Could you check a few things on this model? Use its own coordinates, in mm. A direction names the side the tool comes from. Round coordinates to 2 decimals unless told otherwise and drop trailing zeros. Loops run counter-clockwise (first coordinate to the right, second up) from the corner with the lowest first, then second, coordinate; pieces in that order, holes last. Notation, with made-up numbers: (-37, 49) -> (-30, 49) arc R12 ccw to (-30, 68) -> close; hole circle Ø6 at (-13, 11). An arc over 180 degrees is marked (long way). One line per item, written item: value.
from build123d import *

# Parameters (mm, degrees)
SKETCH1_R                  = 1.1
SKETCH1_W                  = 3
SKETCH1_H                  = 5
SKETCH1_W_2                = 6
SKETCH1_H_2                = 8
BOSS_EXTRUDE1_DEPTH        = 6
F_1_6_1_6_DIAMETER_HOLE3_D = 1.6
BOSS_EXTRUDE2_DEPTH        = 6
FILLET1_R                  = 2
F_2_2_2_2_DIAMETER_HOLE1_D = 2.2
F_4_0MM_DOWEL_HOLE1_D      = 4.5


with BuildPart() as part:
    # Sketch1 → Boss-Extrude1 (new body)
    with BuildSketch(Plane(origin=(0, 0, 0), x_dir=(1, 0, 0), z_dir=(0, 1, 0))):
        Polygon((14.366669751, 50.883801944), (36.883330249, 37.883801944), (36.883330249, -37.883801944), (14.366669751, -50.883801944), (5.706415713, -45.883801944), (5.706415713, -28), (-25.269237886, -28), (-51.25, -13), (-51.25, 13), (-25.269237886, 28), (5.706415713, 28), (5.706415713, 45.883801944), align=None)
        with Locations(Location((14.205771366, 42.605117767, 0), (0, 0, 270))):
            Circle(SKETCH1_R, mode=Mode.SUBTRACT)
        with Locations(Location((29.794228634, 33.605117767, 0), (0, 0, 270))):
            Circle(SKETCH1_R, mode=Mode.SUBTRACT)
        with Locations(Location((29.794228634, -33.605117767, 0), (0, 0, 270))):
            Circle(SKETCH1_R, mode=Mode.SUBTRACT)
        with Locations(Location((14.205771366, -42.605117767, 0), (0, 0, 270))):
            Circle(SKETCH1_R, mode=Mode.SUBTRACT)
        with Locations(Location((-44, 9, 0), (0, 0, 270))):
            Circle(SKETCH1_R, mode=Mode.SUBTRACT)
        with Locations(Location((-44, -9, 0), (0, 0, 270))):
            Circle(SKETCH1_R, mode=Mode.SUBTRACT)
        with BuildLine():
            Line((4.75, -20), (-15.25, -20))
            Line((-15.25, -20), (-15.25, -22))
            Line((-15.25, -22), (-27.25, -22))
            ThreePointArc((-27.25, -22), (-29.75, -19.5), (-27.25, -17))
            Line((-27.25, -17), (-17.25, -17))
            Line((-17.25, -17), (-17.25, 20))
            Line((-17.25, 20), (4.75, 20))
            Line((4.75, 20), (4.75, -20))
        make_face(mode=Mode.SUBTRACT)
        Polygon((30.071152423, 40.084763838), (34.401279442, 37.584763838), (32.901279442, 34.986687627), (28.571152423, 37.486687627), align=None, mode=Mode.SUBTRACT)
        Polygon((15.348720558, 48.584763838), (13.848720558, 45.986687627), (18.178847577, 43.486687627), (19.678847577, 46.084763838), align=None, mode=Mode.SUBTRACT)
        Polygon((34.401279442, -37.584763838), (32.901279442, -34.986687627), (28.571152423, -37.486687627), (30.071152423, -40.084763838), align=None, mode=Mode.SUBTRACT)
        Polygon((18.178847577, -43.486687627), (19.678847577, -46.084763838), (15.348720558, -48.584763838), (13.848720558, -45.986687627), align=None, mode=Mode.SUBTRACT)
        with Locations((-48.25, -8.5)):
            Rectangle(SKETCH1_W, SKETCH1_H, mode=Mode.SUBTRACT)
        with Locations((-48.25, 8.5)):
            Rectangle(SKETCH1_W, SKETCH1_H, mode=Mode.SUBTRACT)
        with BuildLine():
            Line((-30.75, 14.5), (-30.75, 17.5))
            ThreePointArc((-30.75, 17.5), (-29.25, 19), (-27.75, 17.5))
            Line((-27.75, 17.5), (-27.75, 14.5))
            ThreePointArc((-27.75, 14.5), (-29.25, 13), (-30.75, 14.5))
        make_face(mode=Mode.SUBTRACT)
        with BuildLine():
            Line((24.206415713, -25), (24.206415713, -22))
            ThreePointArc((24.206415713, -22), (25.706415713, -20.5), (27.206415713, -22))
            Line((27.206415713, -22), (27.206415713, -25))
            ThreePointArc((27.206415713, -25), (25.706415713, -26.5), (24.206415713, -25))
        make_face(mode=Mode.SUBTRACT)
        with BuildLine():
            Line((24.206415713, 22), (24.206415713, 25))
            ThreePointArc((24.206415713, 25), (25.706415713, 26.5), (27.206415713, 25))
            Line((27.206415713, 25), (27.206415713, 22))
            ThreePointArc((27.206415713, 22), (25.706415713, 20.5), (24.206415713, 22))
        make_face(mode=Mode.SUBTRACT)
        with Locations((29.633330249, 0)):
            Rectangle(SKETCH1_W_2, SKETCH1_H_2, mode=Mode.SUBTRACT)
    extrude(amount=BOSS_EXTRUDE1_DEPTH)

    # Ø1.6 (1.6) Diameter Hole3 (through all)
    with Locations(Plane(origin=(-6.25, 0, 22.5), x_dir=(0, 0, -1), z_dir=(0, -1, 0))):
        with Locations((0, 0), (45, 0)):
            Hole(F_1_6_1_6_DIAMETER_HOLE3_D / 2)

    # Sketch9 → Boss-Extrude2 (add)
    with BuildSketch(Plane.XZ):
        with BuildLine():
            Line((36.883330249, -9), (36.883330249, -15))
            ThreePointArc((36.883330249, -15), (38.383330249, -14.598076211), (39.481406461, -13.5))
            ThreePointArc((39.481406461, -13.5), (39.883330249, -12), (39.481406461, -10.5))
            ThreePointArc((39.481406461, -10.5), (38.383330249, -9.401923789), (36.883330249, -9))
        make_face()
        with BuildLine():
            Line((36.883330249, -6), (36.883330249, -9))
            ThreePointArc((36.883330249, -9), (38.383330249, -9.401923789), (39.481406461, -10.5))
            Line((39.481406461, -10.5), (36.883330249, -6))
        make_face()
        with BuildLine():
            Line((36.883330249, -15), (36.883330249, -18))
            Line((36.883330249, -18), (39.481406461, -13.5))
            ThreePointArc((39.481406461, -13.5), (38.383330249, -14.598076211), (36.883330249, -15))
        make_face()
        with BuildLine():
            ThreePointArc((39.481406461, 10.5), (39.883330249, 12), (39.481406461, 13.5))
            ThreePointArc((39.481406461, 13.5), (38.383330249, 14.598076211), (36.883330249, 15))
            Line((36.883330249, 15), (36.883330249, 9))
            ThreePointArc((36.883330249, 9), (38.383330249, 9.401923789), (39.481406461, 10.5))
        make_face()
        with BuildLine():
            Line((36.883330249, 6), (39.481406461, 10.5))
            ThreePointArc((39.481406461, 10.5), (38.383330249, 9.401923789), (36.883330249, 9))
            Line((36.883330249, 9), (36.883330249, 6))
        make_face()
        with BuildLine():
            ThreePointArc((36.883330249, 15), (38.383330249, 14.598076211), (39.481406461, 13.5))
            Line((39.481406461, 13.5), (36.883330249, 18))
            Line((36.883330249, 18), (36.883330249, 15))
        make_face()
    extrude(amount=-BOSS_EXTRUDE2_DEPTH)

    # Fillet1
    fillet1_edges = [part.edges().sort_by_distance(p)[0] for p in [
        (32.633330249, 3, 4),
        (32.633330249, 3, -4),
        (26.633330249, 3, -4),
        (26.633330249, 3, 4),
    ]]
    fillet(fillet1_edges, radius=FILLET1_R)

    # Ø2.2 (2.2) Diameter Hole1 (through all)
    with Locations(Plane(origin=(20.133330249, 6, -12), x_dir=(0, 0, 1), z_dir=(0, 1, 0))):
        with Locations((0, 0), (24, 0)):
            Hole(F_2_2_2_2_DIAMETER_HOLE1_D / 2)

    # Ø4.0mm Dowel Hole1 (through all)
    with Locations(Plane(origin=(31.883330249, 6, -12), x_dir=(0, 0, 1), z_dir=(0, 1, 0))):
        with Locations((0, 0), (24, 0)):
            Hole(F_4_0MM_DOWEL_HOLE1_D / 2)


solid = part.part
(1) If we section it at C-C, the plane y = 4.55: Give the number of separate pieces and of enclosed holes in the cut face, then the cut area to 3 significant figures.
Recorded:
separate pieces: 1
enclosed holes: 23
area: 4,480 mm²
(2) For faces 1 (the face through (-5, 3, 20)), 2 (the face through (38.2, 2.96, -8.28)), 3 (the face through (-51.25, 3, 0)), which set-ups out of +Z, -Z, +X, -X, +Y, -Y let a thin tool reach every point of the face, with its end or its side?
Recorded:
face 1: +Y, -Y
face 2: +X, +Y, -Y
face 3: +Z, -Z, -X, +Y, -Y
(3) If we section it at B-B, the plane z = -30: Please give me the cut outline in (x, y), then the cut area to 3 significant figures.
Recorded:
outline: (5.71, 0) -> (36.88, 0) -> (36.88, 6) -> (5.71, 6) -> close
area: 187 mm²
(4) If we section it at A-A, the plane x = -22: Please give me the cut outline in (y, z), then the cut area to 3 significant figures.
Recorded:
outline: (0, -28) -> (6, -28) -> (6, 17) -> (0, 17) -> close; (0, 22) -> (6, 22) -> (6, 28) -> (0, 28) -> close
area: 306 mm²
(5) If I drill on L1, parallel to X at y = 2.6, z = -12; L2, parallel to Z at x = 4, y = 5.3; L3, parallel to X at y = 3.4, z = -0.5, over which ranges is the centre line in solid material (lowest first)?
Recorded:
L1: -51.25 to -17.25, 4.75 to 19.03, 21.23 to 29.63, 34.13 to 39.88
L2: -28 to -20, 20 to 28
L3: -51.25 to -17.25, 4.75 to 26.63, 32.63 to 36.88
(6) If we section it at D-D, the plane x = -34.5: Please give me the cut outline in (y, z).
Recorded:
outline: (0, -22.67) -> (6, -22.67) -> (6, 22.67) -> (0, 22.67) -> close
(7) Thinking about a two-plate mould opening in Z: for faces 4 (the face through (-22, 3, 17)), 5 (the face through (5.706, 3, 37)), which applies, released by +Z, released by -Z, zero draft, split by the parting line, or undercut?
Recorded:
face 4: undercut
face 5: zero draft
(8) I'm going to push flat-ended pins straight in: pin 1 Ø3 at (y, z) = (2.5, -1.5) entering from +X; pin 2 Ø2 at (x, y) = (29.5, 4) entering from -Z; pin 3 Ø1.6 at (y, z) = (3.5, 21.5) entering from -X. Where does each tip first touch, or does it pass through?
Recorded:
pin 1: x = 36.88
pin 2: z = -42.72
pin 3: x = -37.91
